Could you check a few things on this drawing? It's one solid part, dimensions in mm from its lowest x, y, z. A direction names the side the tool comes from. Give positions to 0.01 mm unless a question says otherwise; leave off trailing zeros. Loops run counter-clockwise (first coordinate to the right, second up) from the corner with the lowest first, then second, coordinate; pieces in that order, holes last. Notation, with made-up numbers: (37, -22) -> (53, -22) arc R34 ccw to (53, 8) -> close; hole circle Ø5 at (-16.75, 41). An arc over 180 degrees is marked (long way). Use CSV: the item, a comma, the result in double quotes.
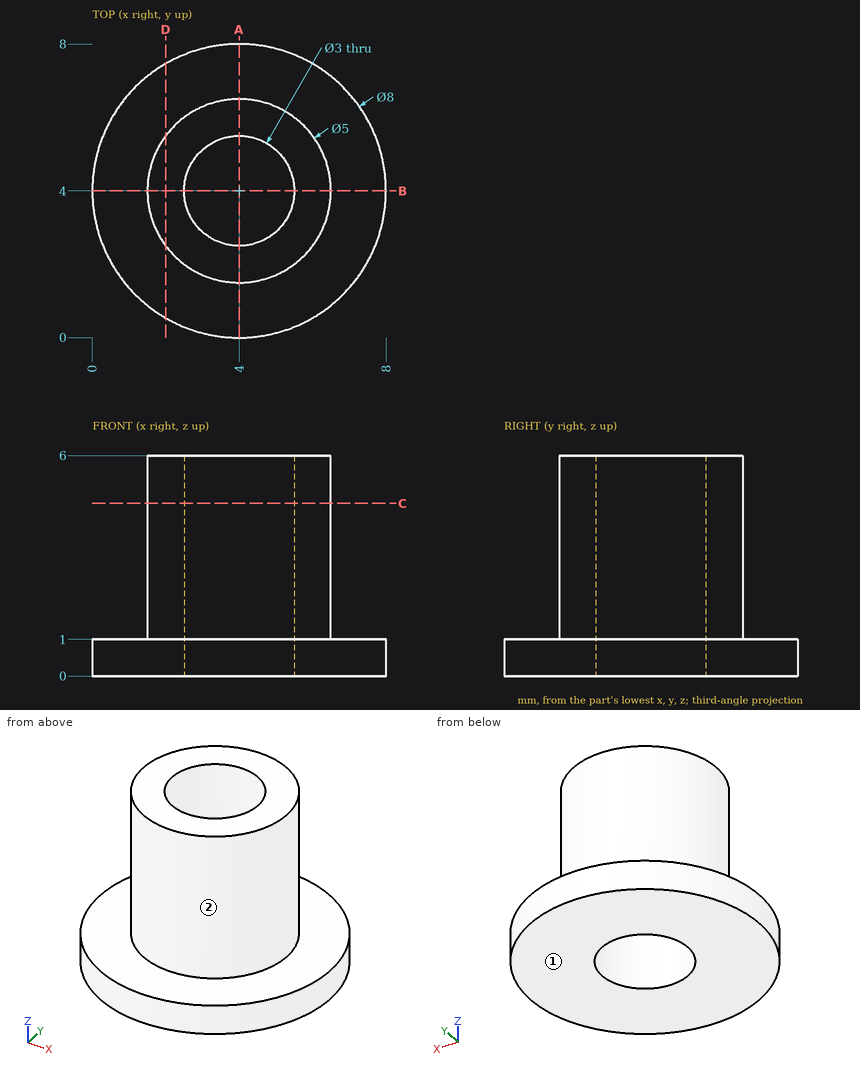
(1) If we section it at C-C, the plane z = 4.7: Write out the boundary of the cut face in (x, y).
Answer sheet:
outline,"circle Ø5 at (4, 4); hole circle Ø3 at (4, 4)"
(2) Which directions (+Z, -Z, +X, -X, +Y, -Y) give clear straight access to the entire face, cutting with the end or side of a thin tool? Please do the marked faces 1 and 2.
Answer sheet:
face 1,"-Z, +X, -X, +Y, -Y"
face 2,"+Z"
(3) If I drill on L1, parallel to Y at x = 4, z = 1.55; L2, parallel to Z at x = 0.75, y = 4.5; L3, parallel to X at y = 5.25, z = 5.25, over which ranges is the centre line in solid material (lowest first)? Write a range as from..to.
Answer sheet:
L1,"y = 1.5..2.5, 5.5..6.5"
L2,"z = 0..1"
L3,"x = 1.83..3.17, 4.83..6.17"
(4) Will this pin go through, and if not, where does the flat tip stop? pin 1 Ø1 at (x, z) = (2, 3.5) entering from +Y.
Answer sheet:
pin 1,"stops at y = 6"
(5) If we section it at D-D, the plane x = 2: Write out the boundary of the cut face in (y, z).
Answer sheet:
outline,"(0.54, 0) -> (7.46, 0) -> (7.46, 1) -> (5.5, 1) -> (5.5, 6) -> (2.5, 6) -> (2.5, 1) -> (0.54, 1) -> close"
(6) If we section it at A-A, the plane x = 4: Write out the boundary of the cut face in (y, z).
Answer sheet:
outline,"(0, 0) -> (2.5, 0) -> (2.5, 6) -> (1.5, 6) -> (1.5, 1) -> (0, 1) -> close; (5.5, 0) -> (8, 0) -> (8, 1) -> (6.5, 1) -> (6.5, 6) -> (5.5, 6) -> close"
